Read the model definition and answer for the solid it produces. Units are mm, in the model's axes. Face numbers are marked on the shaded views. A direction names the side the tool comes from. Give positions to 0.01 mm unless a question says otherwise; leave off trailing zeros. Order: outer loops, then holes, each group sorted by start corner. A loop starts at its lowest first (then second) coordinate and runs counter-clockwise, first axis right, second up. Notation, with made-up numbers: (39.25, 31.5) -> (46.25, 31.5) arc R6 cw to (46.25, 41.5) -> close; hole circle Ø8 at (77.5, 5). An arc over 180 degrees is marked (long way). Answer as CSV lines item,"result". Start each with the question number.
1) The mould has two halves that part along X. Classify the marked faces 1, 2 and 3: +X half, -X half, draft (parallel to the pull), parting line (faces both ways), or undercut.
2) Straight lines are drawn through the part: L1, parallel to Y at x = 0, z = 5.25; L2, parallel to Y at x = -0.5, z = 3.75; L3, parallel to Y at x = 5.5, z = 6. For each, find the intervals that lie inside material, in ascending order. Write a range as from..to.
3) Find section C-C (x = -7). Determine the outline of the cut face in (y, z) (3 decimals), and give its area (3 significant figures).
4) Find section A-A (x = 0). Determine the outline of the cut face in (y, z), and give its area (3 significant figures).
5) For the marked faces 4 and 5, determine the directions among +Z, -Z, +X, -X, +Y, -Y from which every point of the face is accessible in a straight line to the end or side of a thin tool.
6) Find section B-B (z = 2). Determine the outline of the cut face in (x, y).
7) Flat-ended cylindrical pins translate along their axes: pin 1 Ø4 at (y, z) = (-13.5, 1.5) entering from +X; pin 2 Ø2 at (y, z) = (12, 6.5) entering from +X; pin 3 Ø5 at (y, z) = (-8.5, 5) entering from -X. Find the tip coordinate at first contact, or state that the pin passes through.
8) Find section D-D (y = 7.5). Determine the outline of the cut face in (x, z).
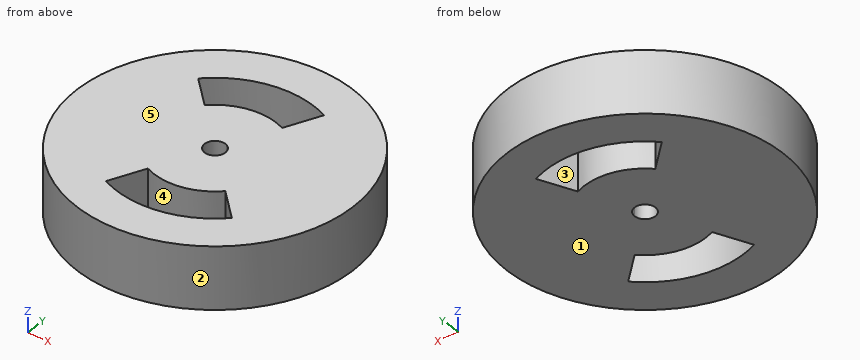
```python
from build123d import *

# Parameters (mm, degrees)
F0_R     = 20
F1_DEPTH = 9


# Not quite as in the source:
# - a feature names something its author has since deleted; it is built from what else it names


with BuildPart() as f1:
    # F0 (on Top) → F1 (new body)
    with BuildSketch(Plane.XY):
        Circle(F0_R)
        with BuildLine():
            Line((-6.0368402564, -13.007011068), (-3.7146515348, -8.0036097652))
            ThreePointArc((-3.7146515348, -8.0036097652), (1.5436452389, -8.6875522833), (6.244462038, -6.2340275228))
            Line((6.244462038, -6.2340275228), (10.1481443029, -10.1311867228))
            ThreePointArc((10.1481443029, -10.1311867228), (2.5086443863, -14.1185155221), (-6.0368402564, -13.007011068))
        make_face(mode=Mode.SUBTRACT)
        with BuildLine():
            Line((6.0368402564, 13.007011068), (3.7146515348, 8.0036097652))
            ThreePointArc((3.7146515348, 8.0036097652), (-1.5436452389, 8.6875522833), (-6.244462038, 6.2340275228))
            Line((-6.244462038, 6.2340275228), (-10.1481443029, 10.1311867228))
            ThreePointArc((-10.1481443029, 10.1311867228), (-2.5086443863, 14.1185155221), (6.0368402564, 13.007011068))
        make_face(mode=Mode.SUBTRACT)
        with BuildLine():
            ThreePointArc((0.6314837286, 1.3605985082), (1.2643626048, 0.8070856234), (1.5, 0))
            ThreePointArc((1.5, 0), (-1.2643626048, -0.8070856234), (0.6314837286, 1.3605985082))
        make_face(mode=Mode.SUBTRACT)
    extrude(amount=F1_DEPTH)


solid = f1.part
```
Findings below:
1,face 1,"draft"
1,face 2,"parting line"
1,face 3,"undercut"
2,L1,"-20..-14.34, -8.82..-1.5, 1.5..8.82, 14.34..20"
2,L2,"-19.99..-14.33, -8.81..-1.41, 1.41..8.81, 14.33..19.99"
2,L3,"-19.23..-13.24, -6.9..11.85, 13.24..19.23"
3,outline,"(-18.735, 0) -> (6.988, 0) -> (6.988, 9) -> (-18.735, 9) -> close; (12.515, 0) -> (18.735, 0) -> (18.735, 9) -> (12.515, 9) -> close"
3,area,"287 mm²"
4,outline,"(-20, 0) -> (-14.34, 0) -> (-14.34, 9) -> (-20, 9) -> close; (-8.82, 0) -> (-1.5, 0) -> (-1.5, 9) -> (-8.82, 9) -> close; (1.5, 0) -> (8.82, 0) -> (8.82, 9) -> (1.5, 9) -> close; (14.34, 0) -> (20, 0) -> (20, 9) -> (14.34, 9) -> close"
4,area,"234 mm²"
5,face 4,"+Z, -Z"
5,face 5,"+Z, +X, -X, +Y, -Y"
6,outline,"circle Ø40 at (0, 0); hole (-10.15, 10.13) -> (-6.24, 6.23) arc R8.82 cw to (3.71, 8) -> (6.04, 13.01) arc R14.34 ccw to start; hole (-6.04, -13.01) arc R14.34 ccw to (10.15, -10.13) -> (6.24, -6.23) arc R8.82 cw to (-3.71, -8) -> close; hole circle Ø3 at (0, 0)"
7,pin 1,"x = 16.36"
7,pin 2,"x = 16.7"
7,pin 3,"x = -19.08"
8,outline,"(-18.54, 0) -> (-7.51, 0) -> (-7.51, 9) -> (-18.54, 9) -> close; (-4.65, 0) -> (18.54, 0) -> (18.54, 9) -> (-4.65, 9) -> close"
